from build123d import *

# Parameters (mm, degrees)
F1_DEPTH = 3.175


with BuildPart() as f1:
    # F0 (on Right) → F1 (new body)
    with BuildSketch(Plane.YZ):
        with BuildLine():
            Line((46.394076, -58.570202), (-144.304461, -58.570202))
            Line((-144.304461, -58.570202), (-144.304461, -75.080202))
            Line((-144.304461, -75.080202), (-147.504861, -75.080202))
            Line((-147.504861, -75.080202), (-147.504861, -58.570202))
            Line((-147.504861, -58.570202), (-312.604861, -58.570202))
            Line((-312.604861, -58.570202), (-312.604861, -78.091796))
            Line((-312.604861, -78.091796), (-315.144861, -78.091796))
            Line((-315.144861, -78.091796), (-315.144861, -87.565996))
            Line((-315.144861, -87.565996), (-86.772296, -87.565996))
            Line((-86.772296, -87.565996), (-86.772296, -72.960996))
            Line((-86.772296, -72.960996), (-83.571896, -72.960996))
            Line((-83.571896, -72.960996), (-83.571896, -87.565996))
            Line((-83.571896, -87.565996), (-82.093418, -87.565996))
            ThreePointArc((-82.093418, -87.565996), (-22.517711, -85.778555), (36.843676, -80.422662))
            Line((36.843676, -80.422662), (36.843676, -68.559073))
            Line((36.843676, -68.559073), (40.044076, -68.559073))
            Line((40.044076, -68.559073), (40.044076, -77.449073))
            Line((40.044076, -77.449073), (46.394076, -77.449073))
            Line((46.394076, -77.449073), (46.394076, -58.570202))
        make_face()
        with BuildLine():
            Line((-54.485447, -83.335202), (-65.48397, -83.335202))
            ThreePointArc((-65.48397, -83.335202), (-68.233601, -81.747702), (-68.233601, -78.572702))
            Line((-68.233601, -78.572702), (-62.734339, -69.047702))
            ThreePointArc((-62.734339, -69.047702), (-59.984709, -67.460202), (-57.235078, -69.047702))
            Line((-57.235078, -69.047702), (-51.735817, -78.572702))
            ThreePointArc((-51.735817, -78.572702), (-51.735817, -81.747702), (-54.485447, -83.335202))
        make_face(mode=Mode.SUBTRACT)
        with BuildLine():
            Line((-40.019661, -78.572702), (-34.520399, -69.047702))
            ThreePointArc((-34.520399, -69.047702), (-31.770769, -67.460202), (-29.021138, -69.047702))
            Line((-29.021138, -69.047702), (-23.521877, -78.572702))
            ThreePointArc((-23.521877, -78.572702), (-23.521877, -81.747702), (-26.271507, -83.335202))
            Line((-26.271507, -83.335202), (-37.27003, -83.335202))
            ThreePointArc((-37.27003, -83.335202), (-40.019661, -81.747702), (-40.019661, -78.572702))
        make_face(mode=Mode.SUBTRACT)
        with BuildLine():
            ThreePointArc((-68.783527, -62.380202), (-66.033896, -63.967702), (-66.033896, -67.142702))
            Line((-66.033896, -67.142702), (-71.533157, -76.667702))
            ThreePointArc((-71.533157, -76.667702), (-74.282788, -78.255202), (-77.032419, -76.667702))
            Line((-77.032419, -76.667702), (-82.53168, -67.142702))
            ThreePointArc((-82.53168, -67.142702), (-82.53168, -63.967702), (-79.782049, -62.380202))
            Line((-79.782049, -62.380202), (-68.783527, -62.380202))
        make_face(mode=Mode.SUBTRACT)
        with BuildLine():
            ThreePointArc((-54.31774, -67.142702), (-54.31774, -63.967702), (-51.568109, -62.380202))
            Line((-51.568109, -62.380202), (-40.569587, -62.380202))
            ThreePointArc((-40.569587, -62.380202), (-37.819956, -63.967702), (-37.819956, -67.142702))
            Line((-37.819956, -67.142702), (-43.319217, -76.667702))
            ThreePointArc((-43.319217, -76.667702), (-46.068848, -78.255202), (-48.818479, -76.667702))
            Line((-48.818479, -76.667702), (-54.31774, -67.142702))
        make_face(mode=Mode.SUBTRACT)
        with BuildLine():
            ThreePointArc((6.607539, -75.255), (6.607539, -78.43), (3.857909, -80.0175))
            Line((3.857909, -80.0175), (-7.140614, -80.0175))
            ThreePointArc((-7.140614, -80.0175), (-9.890245, -78.43), (-9.890245, -75.255))
            Line((-9.890245, -75.255), (-4.390983, -65.73))
            ThreePointArc((-4.390983, -65.73), (-1.641353, -64.1425), (1.108278, -65.73))
            Line((1.108278, -65.73), (6.607539, -75.255))
        make_face(mode=Mode.SUBTRACT)
        with BuildLine():
            ThreePointArc((-26.1038, -67.142702), (-26.1038, -63.967702), (-23.354169, -62.380202))
            Line((-23.354169, -62.380202), (-12.355647, -62.380202))
            ThreePointArc((-12.355647, -62.380202), (-9.606016, -63.967702), (-9.606016, -67.142702))
            Line((-9.606016, -67.142702), (-15.105277, -76.667702))
            ThreePointArc((-15.105277, -76.667702), (-17.854908, -78.255202), (-20.604539, -76.667702))
            Line((-20.604539, -76.667702), (-26.1038, -67.142702))
        make_face(mode=Mode.SUBTRACT)
        with BuildLine():
            ThreePointArc((6.323311, -67.142702), (6.323311, -63.967702), (9.072942, -62.380202))
            Line((9.072942, -62.380202), (20.071464, -62.380202))
            ThreePointArc((20.071464, -62.380202), (22.821095, -63.967702), (22.821095, -67.142702))
            Line((22.821095, -67.142702), (17.321834, -76.667702))
            ThreePointArc((17.321834, -76.667702), (14.572203, -78.255202), (11.822572, -76.667702))
            Line((11.822572, -76.667702), (6.323311, -67.142702))
        make_face(mode=Mode.SUBTRACT)
    extrude(amount=F1_DEPTH)


solid = f1.part
CAD build for the part. Positions are in the model's coordinates, mm. A direction names the side the tool comes from. Give positions to 0.01 mm unless a question says otherwise; leave off trailing zeros. Answer in a Markdown table with one row per item. Add a question column.
Item 1: Band-saw the part on A-A on x = 1.95. Give the number of separate pieces and of enclosed holes in the cut face, then the cut area to 3 significant figures.
Item 2: Drop flat-ended pins along their axis: P1, Ø1.6, axis at x = 2.5, y = -17, coming from the -Z side; P2, Ø0.8, axis at x = 1.5, y = -314.5, coming from the +Z side; P3, Ø1, axis at x = 1.5, z = -64, coming from the -Y side. Give the stop position or say it passes through.
Item 3: Mould opens along Z. For faces 3 (the face through (1.57, -23.35, -85.83)), 4 (the face through (1.57, -7.18, -70.56)), 5 (the face through (3.175, -137, -73)) say: +Z half, -Z half, draft (parallel to the pull), parting line (faces both ways), or undercut.
Item 4: Tool access for faces 1 (the face through (1.6, -23.3, -72)), 2 (the face through (0, -137, -73)): list every direction of +Z, -Z, +X, -X, +Y, -Y with a clear straight run to the whole face (end or side of a thin tool).
Item 5: Probe probe 1 along Y at (x, z) = (0.5, -64); probe 2 along Y at (x, z) = (0.95, -78.75); probe 3 along Z at (x, y) = (1.5, -52.5). List the from-to ranges inside material, lowest first.
Reply:
| question | item | result |
|---|---|---|
| 1 | separate pieces | 1 |
| 1 | enclosed holes | 7 |
| 1 | area | 8,600 mm^2 |
| 2 | P1 | stops at z = -85.48 |
| 2 | P2 | stops at z = -78.09 |
| 2 | P3 | stops at y = -312.6 |
| 3 | face 3 | -Z half |
| 3 | face 4 | undercut |
| 3 | face 5 | draft |
| 4 | face 1 | +X, -X |
| 4 | face 2 | +Z, -Z, -X, +Y, -Y |
| 5 | probe 1 | y = -312.6 to -147.5, -144.3 to -82.55, -66.02 to -54.34, -37.8 to -26.12, -9.59 to 6.3, 22.84 to 46.39 |
| 5 | probe 2 | y = -315.14 to -86.77, -83.57 to -68.33, -51.64 to -40.11, -23.43 to -9.68, 6.4 to 36.84 |
| 5 | probe 3 | z = -87.13 to -82.64, -77.25 to -70.29, -62.52 to -58.57 |
